Answer from the drawing. Dimensions are ordinates in mm from the lowest x, y and z of the part. A direction names the side the tool comes from. Coordinates: 2 decimals unless noted, no trailing zeros. Loops run counter-clockwise (first coordinate to the right, second up) from the corner with the lowest first, then second, coordinate; pieces in that order, holes last.
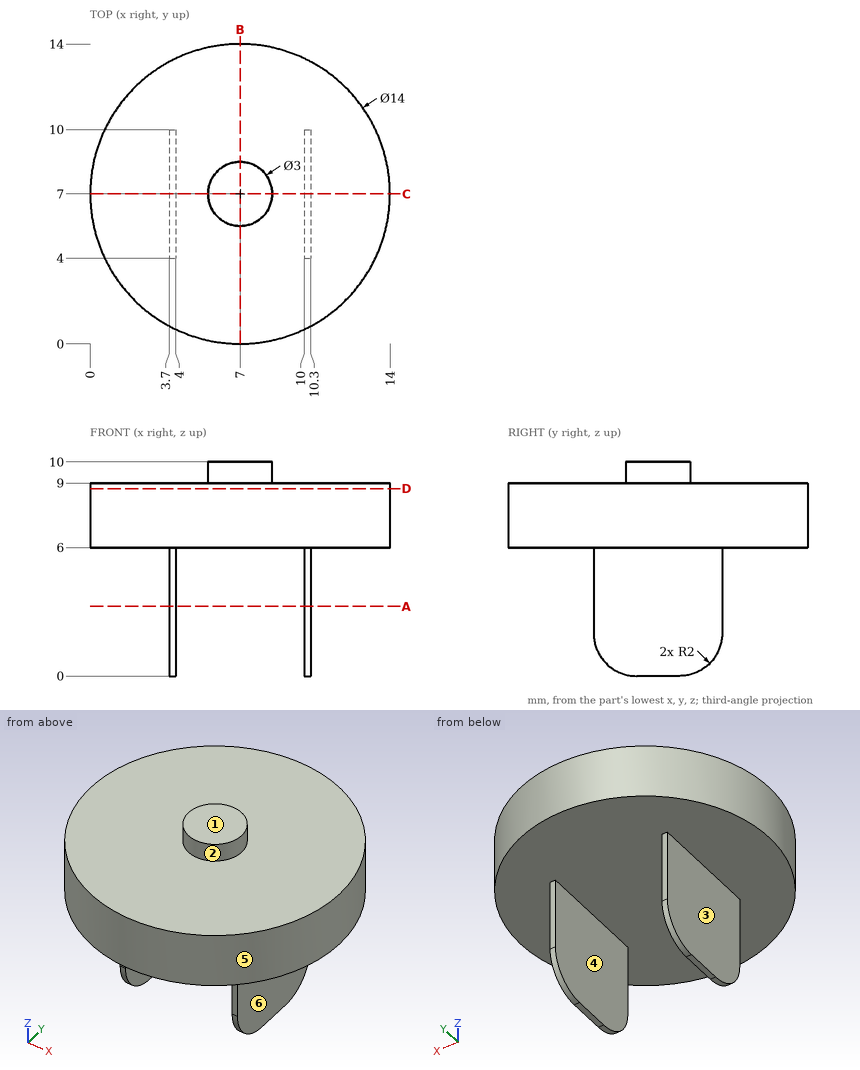
Item 1: A cutting plane is placed at C-C on y = 7. Determine the outline of the cut face in (x, z), then the cut area to 3 significant figures.
Numbers:
outline: (0, 6) - (3.7, 6) - (3.7, 0) - (4, 0) - (4, 6) - (10, 6) - (10, 0) - (10.3, 0) - (10.3, 6) - (14, 6) - (14, 9) - (8.5, 9) - (8.5, 10) - (5.5, 10) - (5.5, 9) - (0, 9) - close
area: 48.6 mm2
Item 2: A cutting plane is placed at B-B on x = 7. Determine the outline of the cut face in (y, z).
Numbers:
outline: (0, 6) - (14, 6) - (14, 9) - (8.5, 9) - (8.5, 10) - (5.5, 10) - (5.5, 9) - (0, 9) - close
Item 3: Given pin 1 (5 mm diameter, centred on x = 6, y = 12.5, fed in from +Z); pin 2 (1 mm diameter, centred on x = 4.5, z = 7.5, fed in from +Y); pin 3 (1.8 mm diameter, centred on y = 7.5, z = 2.5, fed in from -X), each flat-ended and moving along its own axis, determine where each tip first touches the part or whether it passes through.
Numbers:
pin 1: stops at z = 9
pin 2: stops at y = 13.71
pin 3: stops at x = 3.7
Item 4: Find the intervals of material crossed by line 1 along X through (y, z) = (5.5, 5.25); line 2 along Z through (x, y) = (2.75, 10); line 3 along X through (y, z) = (2.5, 8.5), in increasing order.
Numbers:
line 1: x = 3.7 to 4, 10 to 10.3
line 2: z = 6 to 9
line 3: x = 1.64 to 12.36
Item 5: A cutting plane is placed at A-A on z = 3.25. Determine the outline of the cut face in (x, y), then the cut area to 3 significant figures.
Numbers:
outline: (3.7, 4) - (4, 4) - (4, 10) - (3.7, 10) - close; (10, 4) - (10.3, 4) - (10.3, 10) - (10, 10) - close
area: 3.60 mm2
Item 6: Determine the mould class of the marked faces 4, 5 and 6 for opening direction X: released by +X, released by -X, zero draft, split by the parting line, or undercut.
Numbers:
face 4: undercut
face 5: split by the parting line
face 6: released by +X
Item 7: A cutting plane is placed at D-D on z = 8.75. Determine the outline of the cut face in (x, y), then the cut area to 3 significant figures.
Numbers:
outline: circle Ø14 at (7, 7)
area: 154 mm2
Item 8: Which of the six approach directions +Z, -Z, +X, -X, +Y, -Y give full straight-line access (tool end or side, diameter ignored) to the marked faces 1, 2 and 3?
Numbers:
face 1: +Z, +X, -X, +Y, -Y
face 2: +Z
face 3: -Z, -X, +Y, -Y
